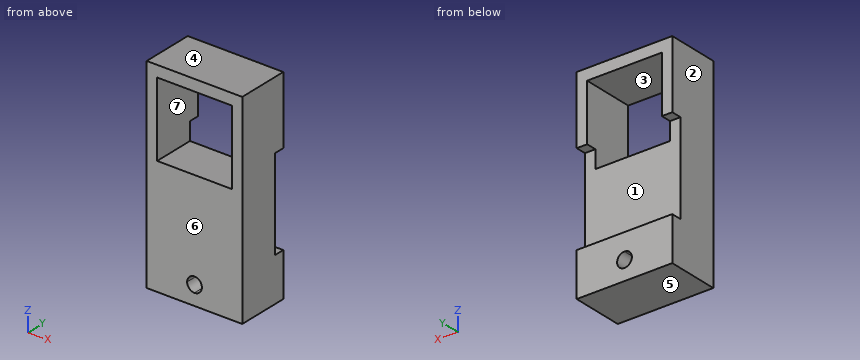
```python
from build123d import *

# Parameters (mm, degrees)
F0_W     = 55
F0_H     = 30
F1_DEPTH = 117
F3_DEPTH = 47.244
F4_W     = 55
F4_H     = 52.50004
F5_DEPTH = 6


with BuildPart() as f1:
    # F0 (on Top) → F1 (new body)
    with BuildSketch(Plane.XY):
        Rectangle(F0_W, F0_H)
    extrude(amount=F1_DEPTH)

    # F2 (on face) → F3 (cut)
    with BuildSketch(Plane(origin=(0, 15, 0), x_dir=(-1, 0, 0), z_dir=(0, 1, 0))):
        with BuildLine():
            ThreePointArc((0, 15.25), (-4.25, 11), (0, 6.75))
            Line((0, 6.75), (0, 11))
            Line((0, 11), (0, 15.25))
        make_face()
        with BuildLine():
            Line((-21.5, 67.5), (0, 67.5))
            Line((0, 67.5), (0, 75))
            ThreePointArc((0, 75), (-14, 89), (0, 103))
            Line((0, 103), (0, 110.5))
            Line((0, 110.5), (-21.5, 110.5))
            Line((-21.5, 110.5), (-21.5, 67.5))
        make_face()
        with BuildLine():
            Line((0, 75), (0, 67.5))
            Line((0, 67.5), (21.5, 67.5))
            Line((21.5, 67.5), (21.5, 110.5))
            Line((21.5, 110.5), (0, 110.5))
            Line((0, 110.5), (0, 103))
            ThreePointArc((0, 103), (9.899495, 98.899495), (14, 89))
            ThreePointArc((14, 89), (9.899495, 79.100505), (0, 75))
        make_face()
        with BuildLine():
            Line((0, 11), (0, 6.75))
            ThreePointArc((0, 6.75), (3.005204, 7.994796), (4.25, 11))
            ThreePointArc((4.25, 11), (3.005204, 14.005204), (0, 15.25))
            Line((0, 15.25), (0, 11))
        make_face()
        with BuildLine():
            ThreePointArc((0, 103), (-14, 89), (0, 75))
            Line((0, 75), (0, 89))
            Line((0, 89), (0, 103))
        make_face()
        with BuildLine():
            Line((0, 89), (0, 75))
            ThreePointArc((0, 75), (9.899495, 79.100505), (14, 89))
            ThreePointArc((14, 89), (9.899495, 98.899495), (0, 103))
            Line((0, 103), (0, 89))
        make_face()
    extrude(amount=-F3_DEPTH, mode=Mode.SUBTRACT)

    # F4 (on face) → F5 (cut)
    with BuildSketch(Plane(origin=(0, 15, 0), x_dir=(-1, 0, 0), z_dir=(0, 1, 0))):
        with Locations((0, 51.5)):
            Rectangle(F4_W, F4_H)
    extrude(amount=-F5_DEPTH, mode=Mode.SUBTRACT)


solid = f1.part
```
Geometry: final body of the model. Coordinates: model frame, mm. Face numbers are marked on the shaded views. A direction names the side the tool comes from. Round coordinates to 2 decimals unless told otherwise and drop trailing zeros. Order: outer loops, then holes, each group sorted by start corner. A loop starts at its lowest first (then second) coordinate and runs counter-clockwise, first axis right, second up. Notation, with made-up numbers: (57, 68) - (105, 68) arc R28 ccw to (105, 95) - close; hole circle Ø7 at (-33, -23). An arc over 180 degrees is marked (long way). Use CSV: the item, a comma, the result in double quotes. Start each with the question number.
Q1. Section query C-C (z = 72.5). Return loops of the section in (x, y), and give its area (3 significant figures).
Q2. Material intervals for line 1 along Z through (x, y) = (4.5, 12.5); line 2 along Z through (x, y) = (13, -10.5); line 3 along X through (y, z) = (12.5, 98), sorted ascending. Write a range as from..to.
Q3. Mould query, pull axis Z, two halves, no side actions, for the marked faces 4, 5, 6 and 7. Classes: +Z half, -Z half, draft (parallel to the pull), parting line (faces both ways), or undercut.
Q4. Section query A-A (y = 13). Return loops of the section in (x, z).
Q5. Section query D-D (x = -23). Return loops of the section in (y, z).
Q6. Section query B-B (x = 20). Return loops of the section in (y, z), and give its area (3 significant figures).
Q7. Access query for the marked faces 1, 2 and 3. Directions: +Z, -Z, +X, -X, +Y, -Y. A direction counts if a zero-diameter tool reaches every point of the face in a straight line with its end or side. Return the directions, or none.
Result set:
1,outline,"(-27.5, -15) - (-21.5, -15) - (-21.5, 9) - (-27.5, 9) - close; (21.5, -15) - (27.5, -15) - (27.5, 9) - (21.5, 9) - close"
1,area,"288 mm2"
2,line 1,"z = 0..25.25, 110.5..117"
2,line 2,"z = 0..67.5, 110.5..117"
2,line 3,"x = -27.5..-21.5, 21.5..27.5"
3,face 4,"+Z half"
3,face 5,"-Z half"
3,face 6,"draft"
3,face 7,"undercut"
4,outline,"(-27.5, 0) - (27.5, 0) - (27.5, 25.25) - (-27.5, 25.25) - close; (-27.5, 77.75) - (-21.5, 77.75) - (-21.5, 110.5) - (21.5, 110.5) - (21.5, 77.75) - (27.5, 77.75) - (27.5, 117) - (-27.5, 117) - close; hole (-4.25, 11) arc R4.25 ccw (long way) to (0, 15.25) arc R4.25 ccw to start"
5,outline,"(-15, 0) - (15, 0) - (15, 25.25) - (9, 25.25) - (9, 77.75) - (15, 77.75) - (15, 117) - (-15, 117) - close"
6,outline,"(-15, 0) - (15, 0) - (15, 25.25) - (9, 25.25) - (9, 67.5) - (-15, 67.5) - close; (-15, 110.5) - (15, 110.5) - (15, 117) - (-15, 117) - close"
6,area,"1,970 mm2"
7,face 1,"+X, -X, +Y"
7,face 2,"+Z, -Z, -X, +Y, -Y"
7,face 3,"+Y, -Y"
